Can you work these out from the model? Positions are in its coordinate system, mm. Face numbers are marked on the shaded views. Round coordinates to 2 decimals unless told otherwise and drop trailing zeros. Order: outer loops, then holes, each group sorted by start corner. A loop starts at its lowest first (then second) coordinate and runs counter-clockwise, first axis right, second up. Notation, with made-up numbers: M -9.75,19.5 L 36.25,19.5 A26 cw 36.25,36.5 Z; hole C 57.25,23.5 d11. An arc over 180 degrees is marked long. One line per question, with ' | ' between items.
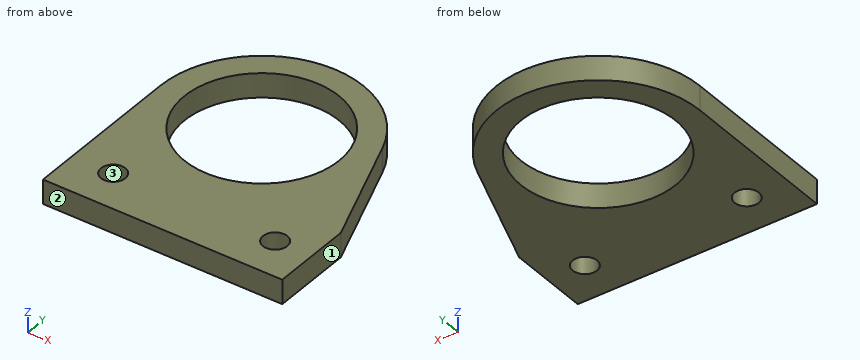
```python
from build123d import *

# Parameters (mm, degrees)
SKETCH_1_R      = 9.55
SKETCH_1_R_2    = 1.5
EXTRUDE_1_DEPTH = 3


with BuildPart() as part:
    # 草图1 → 凸台-拉伸1 (new body)
    with BuildSketch(Plane.XY):
        with BuildLine():
            Line((-12.55, -20), (17, -20))
            Line((17, -20), (17, -10.013370909))
            Line((17, -10.013370909), (11.793142391, 4.292352799))
            ThreePointArc((11.793142391, 4.292352799), (-2.17928463, 12.3593373), (-12.55, 0))
            Line((-12.55, 0), (-12.55, -20))
        make_face()
        Circle(SKETCH_1_R, mode=Mode.SUBTRACT)
        with Locations((-7.5, -15)):
            Circle(SKETCH_1_R_2, mode=Mode.SUBTRACT)
        with Locations((12.5, -15)):
            Circle(SKETCH_1_R_2, mode=Mode.SUBTRACT)
    extrude(amount=EXTRUDE_1_DEPTH)


solid = part.part
```
(1) If we section it at C-C on z = 1.95: Please give me the cut outline in (x, y).
Final values:
outline: M -12.55,-20 L 17,-20 L 17,-10.01 L 11.79,4.29 A12.55 ccw -12.55,0 Z; hole C 0,0 d19.1; hole C -7.5,-15 d3; hole C 12.5,-15 d3
(2) If we section it at A-A on y = 2.5: Please give me the cut outline in (x, z), plus the area to 3 significant figures.
Final values:
outline: M -12.3,0 L -9.22,0 L -9.22,3 L -12.3,3 Z; M 9.22,0 L 12.45,0 L 12.45,3 L 9.22,3 Z | area: 18.9 mm^2
(3) Thinking about a two-plate mould opening in Y: for the marked faces 1, 2 and 3, which applies, released by +Y, released by -Y, zero draft, split by the parting line, or undercut?
Final values:
face 1: zero draft | face 2: released by -Y | face 3: undercut
(4) Please list where these lines run through material, in increasing order: probe 1 along Y at (x, z) = (0, 2.45); probe 2 along Y at (x, z) = (-7, 1.3); probe 3 along X at (y, z) = (-15.5, 2.35). Write a range as [from, to].
Final values:
probe 1: [-20, -9.55], [9.55, 12.55] | probe 2: [-20, -16.41], [-13.59, -6.5], [6.5, 10.42] | probe 3: [-12.55, -8.91], [-6.09, 11.09], [13.91, 17]
(5) If we section it at B-B on x = 0: Please give me the cut outline in (y, z), plus the area to 4 significant figures.
Final values:
outline: M -20,0 L -9.55,0 L -9.55,3 L -20,3 Z; M 9.55,0 L 12.55,0 L 12.55,3 L 9.55,3 Z | area: 40.35 mm^2
(6) If we section it at D-D on x = -7.5: Please give me the cut outline in (y, z), plus the area to 3 significant figures.
Final values:
outline: M -20,0 L -16.5,0 L -16.5,3 L -20,3 Z; M -13.5,0 L -5.91,0 L -5.91,3 L -13.5,3 Z; M 5.91,0 L 10.06,0 L 10.06,3 L 5.91,3 Z | area: 45.7 mm^2
(7) Will these pins go through, and if not, where does the flat tip stop? pin 1 Ø1 at (y, z) = (-5, 2) entering from +X; pin 2 Ø1.5 at (y, z) = (7, 2) entering from -X.
Final values:
pin 1: x = 15.36 | pin 2: x = -10.88
